For this review, take the finished solid that the model builds, in its own axes (mm). Face numbers are marked on the shaded views. A direction names the side the tool comes from. Give positions to 0.01 mm unless a question says otherwise; leave off trailing zeros. Loops run counter-clockwise (first coordinate to the right, second up) from the corner with the lowest first, then second, coordinate; pieces in that order, holes last. Notation, with made-up numbers: (69.5, 69) - (126.5, 69) arc R6 ccw to (126.5, 78) - close; hole circle Ø6 at (59, 13). An arc over 180 degrees is marked (long way). Put each result on its own line as item: value.
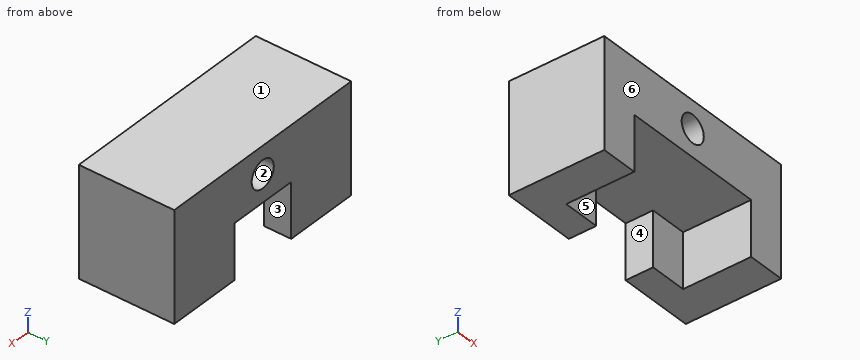
from build123d import *

# Parameters (mm, degrees)
SKETCH1_R           = 1.75
BOSS_EXTRUDE1_DEPTH = 8.7
BOSS_EXTRUDE2_START = 8.7
SKETCH1_3_R         = 1.75
BOSS_EXTRUDE2_DEPTH = 3.5


with BuildPart() as part:
    # Sketch1 → Boss-Extrude1 (new body)
    with BuildSketch(Plane(origin=(0, 0, 0), x_dir=(1, 0, 0), z_dir=(0, 1, 0))):
        Polygon((-9.25, 7), (-14, 7), (-14, -7), (14, -7), (14, 7), (9.25, 7), (9.25, 0), (4.5, 0), (-4.5, 0), (-9.25, 0), align=None)
        with Locations((0, -3.5)):
            Circle(SKETCH1_R, mode=Mode.SUBTRACT)
    extrude(amount=BOSS_EXTRUDE1_DEPTH)

    # Sketch1<3> → Boss-Extrude2 (add)
    with BuildSketch(Plane(origin=(0, 0, 0), x_dir=(1, 0, 0), z_dir=(0, 1, 0)).offset(BOSS_EXTRUDE2_START)):
        Polygon((-14, 7), (-4.5, 7), (-4.5, 0), (4.5, 0), (4.5, 7), (14, 7), (14, -7), (-14, -7), align=None)
        with Locations((0, -3.5)):
            Circle(SKETCH1_3_R, mode=Mode.SUBTRACT)
    extrude(amount=BOSS_EXTRUDE2_DEPTH)


solid = part.part
1) Take a section at B-B on z = -2.75. State the section outline as (x, y) points.
Geometry check:
outline: (-14, 0) - (-9.25, 0) - (-9.25, 8.7) - (-4.5, 8.7) - (-4.5, 12.2) - (-14, 12.2) - close; (4.5, 8.7) - (9.25, 8.7) - (9.25, 0) - (14, 0) - (14, 12.2) - (4.5, 12.2) - close
2) Draft analysis for pull direction Z (two halves, no side actions). For the marked faces 1, 2 and 3, state which applies: pulls with the +Z half, pulls with the -Z half, needs draft (parallel to the pull), parting line crosses it, or undercut.
Geometry check:
face 1: pulls with the +Z half
face 2: undercut
face 3: needs draft
3) Take a section at D-D on z = 3.5. State the section outline as (x, y) points, and give its area (3 significant figures).
Geometry check:
outline: (-14, 0) - (-1.75, 0) - (-1.75, 12.2) - (-14, 12.2) - close; (1.75, 0) - (14, 0) - (14, 12.2) - (1.75, 12.2) - close
area: 299 mm²
4) Take a section at C-C on y = 10. State the section outline as (x, z) points.
Geometry check:
outline: (-14, -7) - (-4.5, -7) - (-4.5, 0) - (4.5, 0) - (4.5, -7) - (14, -7) - (14, 7) - (-14, 7) - close; hole circle Ø3.5 at (0, 3.5)
5) Take a section at A-A on x = 0. State the section outline as (y, z) points.
Geometry check:
outline: (0, 0) - (12.2, 0) - (12.2, 1.75) - (0, 1.75) - close; (0, 5.25) - (12.2, 5.25) - (12.2, 7) - (0, 7) - close
6) Wall thickness on line 1 (X direction, y = 8.5, z = 3.5); line 2 (X direction, y = 2, z = -3); line 3 (Z direction, x = 0, y = 5.25): over which ranges is each line inside the solid? List them lowest first.
Geometry check:
line 1: x = -14 to -1.75, 1.75 to 14
line 2: x = -14 to -9.25, 9.25 to 14
line 3: z = 0 to 1.75, 5.25 to 7
7) Insertion check: pin 1 Ø3.5 at (x, y) = (-2.5, 4.5) entering from -Z. The pin has a flat end and moves straight along its axis. Give the tip position at first contact, or say it passes through.
Geometry check:
pin 1: stops at z = 0
8) For the marked faces 4, 5 and 6, list the 3-axis set-ups (+Z, -Z, +X, -X, +Y, -Y) from which the entire face can be reached by the end or side of a thin tool; tool diameter is ignored.
Geometry check:
face 4: -Z, +Y, -Y
face 5: -Z, -Y
face 6: +Z, -Z, +X, -X, -Y
